```python
from build123d import *

# Parameters (mm, degrees)
F2_R     = 10.5
F3_DEPTH = 110


with BuildPart() as f1:
    # F0 (on Front) → F1 (revolve)
    with BuildSketch(Plane.XZ):
        with BuildLine():
            Line((170, 0), (0, 0))
            Line((0, 0), (0, -24.689806))
            Line((0, -24.689806), (25, -26))
            Line((25, -26), (152, -26))
            ThreePointArc((152, -26), (161.700432, -24.122637), (170, -18.761663))
            Line((170, -18.761663), (170, 0))
        make_face()
    revolve(axis=Axis((85, 0, 0), (1, 0, 0)))

    # F2 (on face) → F3 (cut)
    with BuildSketch(Plane(origin=(0, 0, 0), x_dir=(0, -1, 0), z_dir=(-1, 0, 0))):
        Circle(F2_R)
    extrude(amount=-F3_DEPTH, mode=Mode.SUBTRACT)

    # F4 (on Front) → F5 (revolve, cut)
    with BuildSketch(Plane.XZ):
        Polygon((110, 0), (116.309036, 0), (110, 10.5), align=None)
    revolve(axis=Axis((113.154518, 0, 0), (1, 0, 0)), mode=Mode.SUBTRACT)


solid = f1.part
```
The model under review builds one solid part; all positions refer to its coordinate system, in mm. Round coordinates to 2 decimals unless told otherwise and drop trailing zeros. Write each loop counter-clockwise with the first axis right and the second up, starting at its lowest first coordinate (ties: lowest second). Pieces come first, ordered by that corner, then holes. Notation, with made-up numbers: M 52,37.25 L 103,37.25 A19 cw 103,73.25 Z; hole C 45.25,68 d10. An arc over 180 degrees is marked long. Use CSV: the item, a comma, the result in double quotes. Start each with the question number.
(1) For line 1 along Y through (x, z) = (86, 0); line 2 along Y through (x, z) = (90, -2), list the stretches that pass through material, from the lowest coordinate up.
(2) The part is to be moulded in two halves that separate along Z. For faces 1 (the face through (54.2, -10, 3.2)), 2 (the face through (89.389, -15.821, 20.633)), 3 (the face through (115.2, 1.8, -0.4)), 4 (the face through (0, -11, 0)), say which applies: +Z half, -Z half, draft (parallel to the pull), parting line (faces both ways), or undercut.
(3) Clearance check with flat-ended pins moving along their axes: P1, Ø12, axis at x = 131.5, z = 19.5, coming from the -Y side; P2, Ø1.5, axis at x = 44.5, y = -13.5, coming from the +Z side; P3, Ø1.5, axis at x = 50, y = 2, coming from the -Z side. State where each tip first meets the part, or that it passes through.
(4) We need section A-A, the plane x = 37. State the section outline as (y, z) points.
(5) We need section B-B, the plane x = 139. State the section outline as (y, z) points, then the cut area to 3 significant figures.
Findings:
1,line 1,"-26 to -10.5, 10.5 to 26"
1,line 2,"-25.92 to -10.31, 10.31 to 25.92"
2,face 1,"undercut"
2,face 2,"parting line"
2,face 3,"undercut"
2,face 4,"draft"
3,P1,"y = -22.22"
3,P2,"z = 22.66"
3,P3,"z = -25.97"
4,outline,"C 0,0 d52; hole C 0,0 d21"
5,outline,"C 0,0 d52"
5,area,"2,120 mm^2"
